Read the model definition and answer for the solid it produces. Units are mm, in the model's axes. A direction names the side the tool comes from. Round coordinates to 2 decimals unless told otherwise and drop trailing zeros. Order: outer loops, then holes, each group sorted by start corner. A loop starts at its lowest first (then second) coordinate and runs counter-clockwise, first axis right, second up. Notation, with made-up numbers: M 89,43 L 132,43 A27 cw 132,79 Z; hole C 29.25,-15 d7. An arc over 180 degrees is marked long. Answer as CSV lines item,"result".
```python
from build123d import *

# Parameters (mm, degrees)
BOSS_EXTRUDE1_DEPTH = 15
BOSS_EXTRUDE2_DEPTH = 10
SKETCH3_R           = 1.55
CUT_EXTRUDE1_DEPTH  = 50.497474683
BOSS_EXTRUDE3_START = 8
SKETCH4_R           = 2.5
SKETCH4_R_2         = 1.55
BOSS_EXTRUDE3_DEPTH = 8
SKETCH5_W           = 15
SKETCH5_H           = 12
BOSS_EXTRUDE4_DEPTH = 23.05
BOSS_EXTRUDE5_DEPTH = 5
SKETCH9_W           = 35
SKETCH9_H           = 20
BOSS_EXTRUDE6_DEPTH = 6
FILLET1_R           = 7
FILLET4_R           = 3
FILLET6_R           = 1


with BuildPart() as part:
    # Sketch1 → Boss-Extrude1 (new body)
    with BuildSketch(Plane.XY):
        Polygon((0, 0), (0, -50), (25, -50), (25, -40), (10, -40), (10, 0), align=None)
    extrude(amount=BOSS_EXTRUDE1_DEPTH)

    # Sketch2 → Boss-Extrude2 (add)
    with BuildSketch(Plane.ZY):
        Polygon((10.25, -59), (10.25, -50), (4.75, -50), (4.75, -59), (2.5, -59), (2.5, -62), (6.725601587, -62), (8.274398413, -62), (12.5, -62), (12.5, -59), align=None)
    extrude(amount=-BOSS_EXTRUDE2_DEPTH)

    # Sketch3 → Cut-Extrude1 (cut, through all)
    with BuildSketch(Plane(origin=(0, -40, 0), x_dir=(1, 0, 0), z_dir=(0, 1, 0))):
        with Locations(Location((17.5, -7.5, 0), (0, 0, 270))):
            Circle(SKETCH3_R)
    extrude(amount=-CUT_EXTRUDE1_DEPTH, mode=Mode.SUBTRACT)

    # Sketch4 → Boss-Extrude3 (add)
    with BuildSketch(Plane(origin=(0, -40, 0), x_dir=(1, 0, 0), z_dir=(0, 1, 0)).offset(BOSS_EXTRUDE3_START)):
        with Locations(Location((17.5, -7.5, 0), (0, 0, 90))):
            Circle(SKETCH4_R)
        with Locations(Location((17.5, -7.5, 0), (0, 0, 270))):
            Circle(SKETCH4_R_2, mode=Mode.SUBTRACT)
    extrude(amount=-BOSS_EXTRUDE3_DEPTH)

    # Sketch5 → Boss-Extrude4 (add)
    with BuildSketch(Plane(origin=(10, 0, 0), x_dir=(0, 0, -1), z_dir=(1, 0, 0))):
        with Locations((-7.5, -6)):
            Rectangle(SKETCH5_W, SKETCH5_H)
    extrude(amount=BOSS_EXTRUDE4_DEPTH)

    # Sketch7 → Boss-Extrude5 (add)
    with BuildSketch(Plane.ZY):
        Polygon((0, 0), (0, -50), (4.75, -50), (4.75, -59), (2.5, -59), (2.5, -62), (12.5, -62), (12.5, -59), (10.25, -59), (10.25, -50), (15, -50), (15, 0), align=None)
    extrude(amount=BOSS_EXTRUDE5_DEPTH)

    # Sketch9 → Boss-Extrude6 (add)
    with BuildSketch(Plane(origin=(33.05, 0, 0), x_dir=(0, 0, -1), z_dir=(1, 0, 0))):
        with Locations((-7.5, -6)):
            Rectangle(SKETCH9_W, SKETCH9_H)
    extrude(amount=BOSS_EXTRUDE6_DEPTH)

    # Fillet1
    fillet1_edges = [part.edges().sort_by_distance(p)[0] for p in [
        (36.05, -16, -10),
        (36.05, 4, -10),
        (36.05, 4, 25),
        (36.05, -16, 25),
    ]]
    fillet(fillet1_edges, radius=FILLET1_R)

    # Fillet4
    fillet4_edges = [part.edges().sort_by_distance(p)[0] for p in [
        (10, -40, 7.5),
        (25, -40, 7.5),
        (25, -50, 7.5),
        (10, -12, 7.5),
        (-5, 0, 7.5),
    ]]
    fillet(fillet4_edges, radius=FILLET4_R)

    # Fillet6
    fillet6_edges = [part.edges().sort_by_distance(p)[0] for p in [
        (33.05, -6, 15),
        (33.05, -12, 7.5),
        (33.05, -6, 0),
        (33.05, 0, 7.5),
    ]]
    fillet(fillet6_edges, radius=FILLET6_R)


solid = part.part
```
Item 1: A cutting plane is placed at A-A, the plane x = 17.5. Determine the outline of the cut face in (y, z).
Ans:
outline,"M -50,0 L -40,0 L -40,5 L -32,5 L -32,5.95 L -50,5.95 Z; M -50,9.05 L -32,9.05 L -32,10 L -40,10 L -40,15 L -50,15 Z; M -12,0 L 0,0 L 0,15 L -12,15 Z"
Item 2: A cutting plane is placed at D-D, the plane z = 1.5. Determine the outline of the cut face in (x, y), and give its area (3 significant figures).
Ans:
outline,"M -5,-50 L 22,-50 A3 ccw 25,-47 L 25,-43 A3 ccw 22,-40 L 13,-40 A3 cw 10,-37 L 10,-15 A3 cw 13,-12 L 32.05,-12 A1 cw 33.05,-13 L 33.05,-16 L 39.05,-16 L 39.05,4 L 33.05,4 L 33.05,1 A1 cw 32.05,0 L -2,0 A3 ccw -5,-3 Z"
area,"1,300 mm2"
Item 3: Flat-ended cylindrical pins translate along their axes: pin 1 (12 mm diameter, centred on y = -25, z = 9.5, fed in from +X); pin 2 (4.5 mm diameter, centred on x = 11, z = 9.5, fed in from +Y); pin 3 (2.5 mm diameter, centred on x = 2.5, y = -53, fed in from -Z); pin 4 (3 mm diameter, centred on x = 7, z = 13.5, fed in from -Y). Find the tip coordinate at first contact, or state that the pin passes through.
Ans:
pin 1,"x = 10"
pin 2,"y = 0"
pin 3,"z = 4.75"
pin 4,"y = -62"
Item 4: A cutting plane is placed at C-C, the plane x = 36.5. Determine the outline of the cut face in (y, z).
Ans:
outline,"M -16,-3 A7 ccw -9,-10 L -3,-10 A7 ccw 4,-3 L 4,18 A7 ccw -3,25 L -9,25 A7 ccw -16,18 Z"
Item 5: Determine the mould class of faces 1 (the face through (36, 4, 8)), 2 (the face through (36, -16, 8)), 3 (the face through (3, -59, 11)), 4 (the face through (36, -6, -10)) for opening direction Y: +Y half, -Y half, draft (parallel to the pull), parting line (faces both ways), or undercut.
Ans:
face 1,"+Y half"
face 2,"-Y half"
face 3,"undercut"
face 4,"draft"
Item 6: A tool of negligible diameter and unlimited length cuts with its end or side. For faces 5 (the face through (3, -59, 4)), 6 (the face through (9.7, -25.3, 15)), 7 (the face through (25, -45, 7)), 8 (the face through (19.94, -35.94, 8.04)), 9 (the face through (19, -32, 9)), from which of +Z, -Z, +X, -X, +Y, -Y can it reach the whole face along a straight path? Write none if from no direction.
Ans:
face 5,"-Z, +X, -X"
face 6,"+Z, -X, +Y, -Y"
face 7,"+Z, -Z, +X, -Y"
face 8,"none"
face 9,"+Z, -Z, +X"
Item 7: Find the intervals of material crossed by probe 1 along X at (y, z) = (-37.25, 7.5); probe 2 along X at (y, z) = (-44, 7.5); probe 3 along Y at (x, z) = (2, 4), in increasing order. Write a range as [from, to].
Ans:
probe 1,"[-5, 10.01], [15, 15.95], [19.05, 20]"
probe 2,"[-5, 15.95], [19.05, 25]"
probe 3,"[-62, -59], [-50, 0]"
